```python
from build123d import *

# Parameters (mm, degrees)
F0_R     = 11.05
F1_DEPTH = 7
F2_R     = 15.35
F2_R_2   = 11.05
F3_DEPTH = 7
F4_R     = 15.35
F4_R_2   = 11.05
F5_DEPTH = 7


with BuildPart() as f1:
    # F0 (on Top) → F1 (new body)
    with BuildSketch(Plane.XY):
        with BuildLine():
            ThreePointArc((10.198039, -11), (13.747192, -6.001225), (15, 0))
            ThreePointArc((15, 0), (13.747192, 6.001225), (10.198039, 11))
            ThreePointArc((10.198039, 11), (5.477226, 13.96424), (0, 15))
            ThreePointArc((0, 15), (-5.477226, 13.96424), (-10.198039, 11))
            ThreePointArc((-10.198039, 11), (-15, 0), (-10.198039, -11))
            ThreePointArc((-10.198039, -11), (-5.477226, -13.96424), (0, -15))
            ThreePointArc((0, -15), (5.477226, -13.96424), (10.198039, -11))
        make_face()
        Circle(F0_R, mode=Mode.SUBTRACT)
        with BuildLine():
            ThreePointArc((0, 15), (5.477226, 13.96424), (10.198039, 11))
            Line((10.198039, 11), (30, 11))
            Line((30, 11), (30, 15))
            Line((30, 15), (0, 15))
        make_face()
        with BuildLine():
            Line((30, -11), (10.198039, -11))
            ThreePointArc((10.198039, -11), (5.477226, -13.96424), (0, -15))
            Line((0, -15), (30, -15))
            Line((30, -15), (30, -11))
        make_face()
        with BuildLine():
            ThreePointArc((-10.198039, 11), (-5.477226, 13.96424), (0, 15))
            Line((0, 15), (-30, 15))
            Line((-30, 15), (-29.986673, 11))
            Line((-29.986673, 11), (-10.198039, 11))
        make_face()
        with BuildLine():
            Line((-30, -15), (0, -15))
            ThreePointArc((0, -15), (-5.477226, -13.96424), (-10.198039, -11))
            Line((-10.198039, -11), (-29.98667, -11))
            Line((-29.98667, -11), (-30, -15))
        make_face()
    extrude(amount=F1_DEPTH)

    # F2 (on face) → F3 (join)
    with BuildSketch(Plane(origin=(-29.949681, 0.099805, 0), x_dir=(-0.003332, -0.999994, 0), z_dir=(-0.999994, 0.003332, 0))):
        with Locations((0, 3.5)):
            Circle(F2_R)
        with Locations((0, 3.5)):
            Circle(F2_R_2, mode=Mode.SUBTRACT)
    extrude(amount=F3_DEPTH)

    # F4 (on face) → F5 (join)
    with BuildSketch(Plane.YZ.offset(30)):
        with Locations((0, 3.5)):
            Circle(F4_R)
        with Locations((0, 3.5)):
            Circle(F4_R_2, mode=Mode.SUBTRACT)
    extrude(amount=F5_DEPTH)


solid = f1.part
```
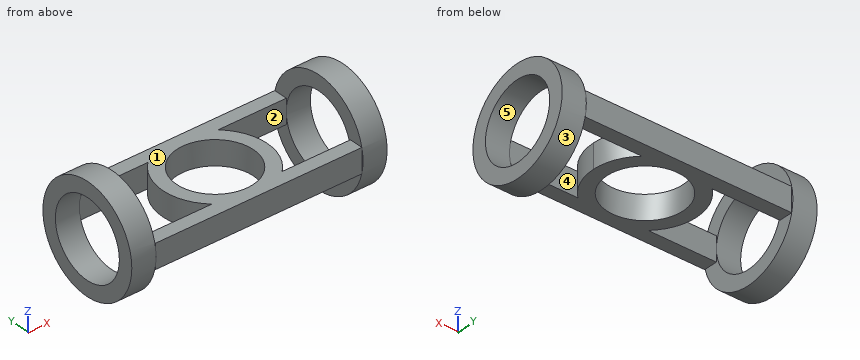
Model file for the job. Use its own axes, mm. Face numbers are marked on the shaded views. A direction names the side the tool comes from. Coordinates: 2 decimals unless noted, no trailing zeros. Write each loop counter-clockwise with the first axis right and the second up, starting at its lowest first coordinate (ties: lowest second). Pieces come first, ordered by that corner, then holes. Notation, with made-up numbers: (15.5, 42) - (33.5, 42) arc R17 cw to (33.5, 62) - close; hole circle Ø8 at (36.25, 15.5). An arc over 180 degrees is marked (long way). Use a Markdown table: item, result. Add a question column.
Item 1: Drop flat-ended pins along their axis: pin 1 (7.5 mm diameter, centred on x = 9, z = 5, fed in from +Y); pin 2 (7.5 mm diameter, centred on x = -15, z = 3.5, fed in from -Y); pin 3 (9 mm diameter, centred on x = 12.5, y = 0, fed in from +Z); pin 4 (8 mm diameter, centred on y = 5.5, z = 13, fed in from +X). Give the stop position or say it passes through.
Item 2: Band-saw the part on A-A, the plane x = 25. Write the cut outline in (y, z).
Item 3: Band-saw the part on B-B, the plane z = 13. Write the cut outline in (x, y).
Item 4: 3-axis set-ups, long thin cutter, end or side, ignore diameter. For the marked faces 1 and 2: which of +Z, -Z, +X, -X, +Y, -Y reach the whole face in a straight line?
Item 5: Two-plate mould, pull along Z, no slides. Class the marked faces 3, 4 and 5: pulls with the +Z half, pulls with the -Z half, needs draft (parallel to the pull), parting line crosses it, or undercut.
Item 6: Band-saw the part on D-D, the plane x = 0. Write the cut outline in (y, z), and give its area (3 significant figures).
Item 7: Drill centre lines: line 1 along Y through (x, z) = (33.5, 3.5); line 2 along X through (y, z) = (-7.5, -7.5) (3 decimals); line 3 along Y through (x, z) = (0, 1). Where is each one in solid material? Low to high.
A:
| question | item | result |
|---|---|---|
| 1 | pin 1 | stops at y = 15 |
| 1 | pin 2 | stops at y = -15 |
| 1 | pin 3 | stops at z = 7 |
| 1 | pin 4 | stops at x = 37 |
| 2 | outline | (-15, 0) - (-11, 0) - (-11, 7) - (-15, 7) - close; (11, 0) - (15, 0) - (15, 7) - (11, 7) - close |
| 3 | outline | (-36.99, -11.93) - (-29.99, -11.96) - (-29.97, -5.54) - (-36.97, -5.52) - close; (-36.93, 5.77) - (-29.93, 5.74) - (-29.91, 12.16) - (-36.91, 12.18) - close; (30, -12.06) - (37, -12.06) - (37, -5.64) - (30, -5.64) - close; (30, 5.64) - (37, 5.64) - (37, 12.06) - (30, 12.06) - close |
| 4 | face 1 | +Z, +Y, -Y |
| 4 | face 2 | +Z, -Z |
| 5 | face 3 | parting line crosses it |
| 5 | face 4 | needs draft |
| 5 | face 5 | undercut |
| 6 | outline | (-15, 0) - (-11.05, 0) - (-11.05, 7) - (-15, 7) - close; (11.05, 0) - (15, 0) - (15, 7) - (11.05, 7) - close |
| 6 | area | 55.3 mm² |
| 7 | line 1 | y = -15.35 to -11.05, 11.05 to 15.35 |
| 7 | line 2 | x = -36.975 to -29.975, 30 to 37 |
| 7 | line 3 | y = -15 to -11.05, 11.05 to 15 |
